from build123d import *

# Parameters (mm, degrees)
SKETCH1_R           = 7
BOSS_EXTRUDE1_DEPTH = 48
SKETCH2_R           = 2.25
BOSS_EXTRUDE2_DEPTH = 1
SKETCH3_R           = 4.5
BOSS_EXTRUDE3_DEPTH = 0.5
SKETCH4_R           = 3
SKETCH4_R_2         = 2.5
CUT_EXTRUDE1_DEPTH  = 1.5


with BuildPart() as part:
    # Sketch1 → Boss-Extrude1 (new body)
    with BuildSketch(Plane(origin=(0, 0, 0), x_dir=(1, 0, 0), z_dir=(0, 1, 0))):
        Circle(SKETCH1_R)
    extrude(amount=BOSS_EXTRUDE1_DEPTH)

    # Sketch2 → Boss-Extrude2 (add)
    with BuildSketch(Plane(origin=(0, 48, 0), x_dir=(1, 0, 0), z_dir=(0, 1, 0))):
        Circle(SKETCH2_R)
    extrude(amount=BOSS_EXTRUDE2_DEPTH)

    # Sketch3 → Boss-Extrude3 (add)
    with BuildSketch(Plane(origin=(0, 0, 0), x_dir=(1, 0, 0), z_dir=(0, 1, 0))):
        Circle(SKETCH3_R)
    extrude(amount=-BOSS_EXTRUDE3_DEPTH)

    # Sketch4 → Cut-Extrude1 (cut, through all)
    with BuildSketch(Plane(origin=(0, 0, 0), x_dir=(1, 0, 0), z_dir=(0, 1, 0))):
        Circle(SKETCH4_R)
        Circle(SKETCH4_R_2, mode=Mode.SUBTRACT)
    extrude(amount=-CUT_EXTRUDE1_DEPTH, mode=Mode.SUBTRACT)


solid = part.part
Geometry: final body of the model. Coordinates: model frame, mm. A direction names the side the tool comes from. Give positions to 0.01 mm unless a question says otherwise; leave off trailing zeros. Loops run counter-clockwise (first coordinate to the right, second up) from the corner with the lowest first, then second, coordinate; pieces in that order, holes last. Notation, with made-up numbers: M 27,-17 L 77,-17 A15 cw 77,12 Z; hole C -7,3 d8. An arc over 180 degrees is marked long. Put each result on its own line as item: value. Start each with the question number.
1) Cut plane A-A (x = 0). Output: boundary loops of the cut face in (y, z).
2) Cut plane B-B (z = 0). Output: boundary loops of the cut face in (x, y).
3) Access query for faces 4 (the flat face through (-2, 48, -2)), 5 (the cylindrical face through (-0.59, -0.25, -4.46)), 6 (the cylindrical face through (6.466, 23.664, 2.681)). Directions: +Z, -Z, +X, -X, +Y, -Y. A direction counts if a zero-diameter tool reaches every point of the face in a straight line with its end or side. Return the directions, or none.
4) Pull-direction query (Z, two-part tool) for faces 1 (the cylindrical face through (-0.29, 48.49, -2.23)), 2 (the cylindrical face through (-3, -0.2, -0.1)), 3 (the flat face through (0, -0.5, 0)); classes: pulls with the +Z half, pulls with the -Z half, needs draft (parallel to the pull), parting line crosses it, or undercut.
5) Cut plane C-C (y = 6). Output: boundary loops of the cut face in (x, z).
6) Cut plane D-D (x = 3.75). Output: boundary loops of the cut face in (y, z).
7) Contact query for flat-ended pins moving along their axis: pin 1 (4 mm diameter, centred on y = 30, z = -2.5, fed in from +X); pin 2 (1 mm diameter, centred on x = -3, y = 24, fed in from +Z); pin 3 (1.5 mm diameter, centred on x = 4, z = -3.5, fed in from +Y). Output: stop coordinate, or through.
8) Ray query, line 1 along Z through (x, y) = (0, -0.1); line 2 along Y through (x, z) = (5, -4.25). Return the intervals inside material, ascending.
Verdict:
1. outline: M -0.5,-4.5 L 0,-4.5 L 0,-7 L 48,-7 L 48,-2.25 L 49,-2.25 L 49,2.25 L 48,2.25 L 48,7 L 0,7 L 0,4.5 L -0.5,4.5 L -0.5,3 L 0,3 L 0,2.5 L -0.5,2.5 L -0.5,-2.5 L 0,-2.5 L 0,-3 L -0.5,-3 Z
2. outline: M -7,0 L -4.5,0 L -4.5,-0.5 L -3,-0.5 L -3,0 L -2.5,0 L -2.5,-0.5 L 2.5,-0.5 L 2.5,0 L 3,0 L 3,-0.5 L 4.5,-0.5 L 4.5,0 L 7,0 L 7,48 L 2.25,48 L 2.25,49 L -2.25,49 L -2.25,48 L -7,48 Z
3. face 4: +Y
3. face 5: -Y
3. face 6: +Y, -Y
4. face 1: parting line crosses it
4. face 2: undercut
4. face 3: needs draft
5. outline: C 0,0 d14
6. outline: M -0.5,-2.49 L 0,-2.49 L 0,-5.91 L 48,-5.91 L 48,5.91 L 0,5.91 L 0,2.49 L -0.5,2.49 Z
7. pin 1: x = 6.98
7. pin 2: z = 6.54
7. pin 3: y = 48
8. line 1: -4.5 to -3, -2.5 to 2.5, 3 to 4.5
8. line 2: 0 to 48
